Input: part model. Units: mm. Frame: model coordinates. A direction names the side the tool comes from. Give positions to 0.01 mm unless a question says otherwise; leave off trailing zeros. Loops run counter-clockwise (first coordinate to the right, second up) from the corner with the lowest first, then second, coordinate; pieces in that order, holes last. Notation, with made-up numbers: M 76.5,67.25 L 113.5,67.25 A20 ccw 113.5,104.25 Z; hole C 83,75 d5. An arc over 180 degrees is marked long. Use a Markdown table: item, result. Add a question column.
from build123d import *

# Parameters (mm, degrees)
F0_W     = 76.2
F0_H     = 213.36
F1_DEPTH = 44.45
F2_T     = -2.54
F3_R     = 2.54


with BuildPart() as f1:
    # F0 (on Top) → F1 (new body)
    with BuildSketch(Plane.XY):
        with Locations((38.1, 106.68)):
            Rectangle(F0_W, F0_H)
    extrude(amount=F1_DEPTH)

    # F2
    f2_openings = [f1.faces().sort_by_distance(p)[0] for p in [
        (38.1, 106.68, 44.45),
    ]]
    offset(amount=F2_T, openings=f2_openings)

    # F3
    f3_edges = [f1.edges().sort_by_distance(p)[0] for p in [
        (0, 0, 22.225),
        (76.2, 0, 22.225),
        (76.2, 213.36, 22.225),
        (0, 213.36, 22.225),
    ]]
    fillet(f3_edges, radius=F3_R)


solid = f1.part
1) Pull-direction query (X, two-part tool) for faces 3 (the flat face through (38, 0, 22)), 4 (the flat face through (0, 105, 22)), 5 (the flat face through (76.2, 105, 22)), 6 (the flat face through (73.66, 105, 23)); classes: pulls with the +X half, pulls with the -X half, needs draft (parallel to the pull), parting line crosses it, or undercut.
2) Ray query, line 1 (X direction, y = 75.5, z = 6.5); line 2 (Y direction, x = 13, z = 9.5); line 3 (Z direction, x = 30.5, y = 161). Return the intervals inside material, ascending. Write a range as [from, to].
3) Section query A-A, the plane z = 40. Return the cut outline in (x, y), and give its area (3 significant figures).
4) Section query C-C, the plane y = 134. Return the cut outline in (x, z).
5) Reachability of faces 1 (the flat face through (38, 2.54, 23)), 2 (the flat face through (38, 213.36, 22)) from +Z, -Z, +X, -X, +Y, -Y: full face, straight path, thin tool, end or side. Return the list, or none.
6) Contact query for a flat-ended pin moving along its axis: P1, Ø21.5, axis at x = 47.5, y = 140.5, coming from the +Z side. Output: stop coordinate, or through.
7) Section query B-B, the plane x = 17.5. Return the cut outline in (y, z), and give its area (3 significant figures).
Entries:
| question | item | result |
|---|---|---|
| 1 | face 3 | needs draft |
| 1 | face 4 | pulls with the -X half |
| 1 | face 5 | pulls with the +X half |
| 1 | face 6 | undercut |
| 2 | line 1 | x = [0, 2.54], [73.66, 76.2] |
| 2 | line 2 | y = [0, 2.54], [210.82, 213.36] |
| 2 | line 3 | z = [0, 2.54] |
| 3 | outline | M 0,2.54 A2.54 ccw 2.54,0 L 73.66,0 A2.54 ccw 76.2,2.54 L 76.2,210.82 A2.54 ccw 73.66,213.36 L 2.54,213.36 A2.54 ccw 0,210.82 Z; hole M 2.54,2.54 L 73.66,2.54 L 73.66,210.82 L 2.54,210.82 Z |
| 3 | area | 1,440 mm² |
| 4 | outline | M 0,0 L 76.2,0 L 76.2,44.45 L 73.66,44.45 L 73.66,2.54 L 2.54,2.54 L 2.54,44.45 L 0,44.45 Z |
| 5 | face 1 | +Z |
| 5 | face 2 | +Z, -Z, +X, -X, +Y |
| 6 | P1 | stops at z = 2.54 |
| 7 | outline | M 0,0 L 213.36,0 L 213.36,44.45 L 210.82,44.45 L 210.82,2.54 L 2.54,2.54 L 2.54,44.45 L 0,44.45 Z |
| 7 | area | 755 mm² |
